Geometry: see drawing. Coordinates: mm, zero at the bounding-box minimum. Round coordinates to 2 decimals unless told otherwise and drop trailing zeros. Order: outer loops, then holes, each group sorted by start corner. A loop starts at its lowest first (then second) coordinate and runs counter-clockwise, first axis right, second up. Notation, with made-up numbers: (88.5, -22) -> (121.5, -22) arc R16 ccw to (121.5, -15) -> close; hole circle Ø11 at (53, 87.25). An arc over 180 degrees is marked (long way). Use a Markdown table: item, result.
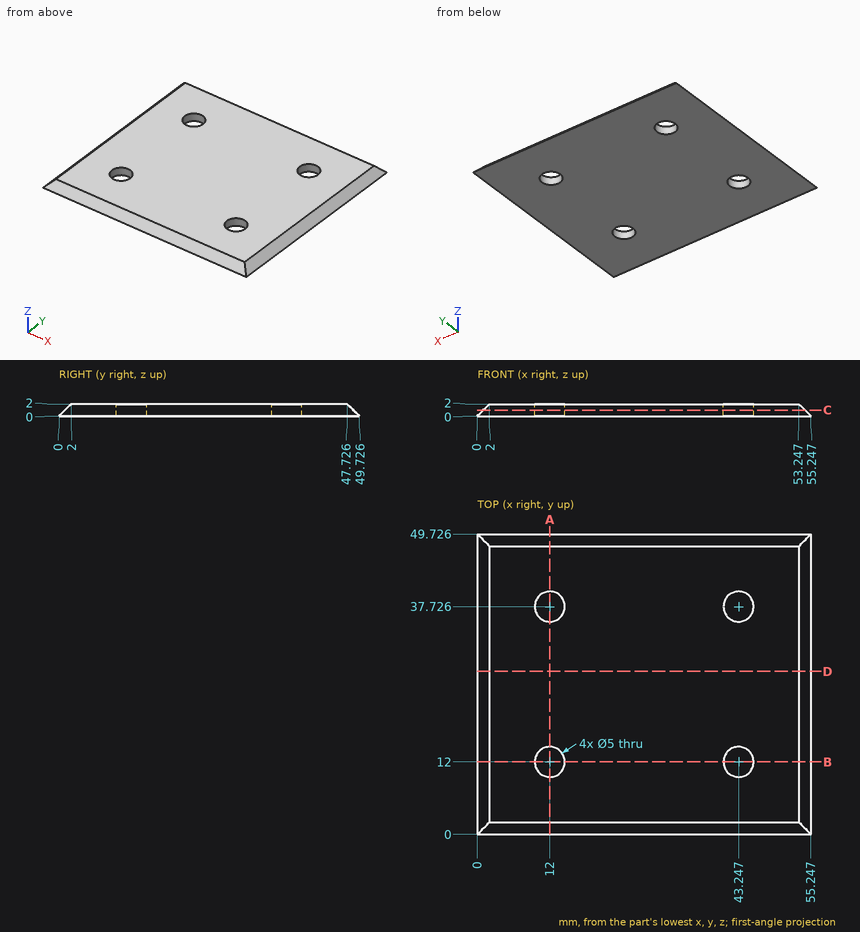
1) Ray query, probe 1 along Y at (x, z) = (12, 1.4) (1 decimal); probe 2 along Y at (x, z) = (12, 1.2) (1 decimal); probe 3 along X at (y, z) = (10, 1.35). Return the intervals inside material, ascending.
Answer key:
| item | result |
|---|---|
| probe 1 | y = 1.4 to 9.5, 14.5 to 35.2, 40.2 to 48.3 |
| probe 2 | y = 1.2 to 9.5, 14.5 to 35.2, 40.2 to 48.5 |
| probe 3 | x = 1.35 to 10.5, 13.5 to 41.75, 44.75 to 53.9 |
2) Cut plane A-A on x = 12. Return loops of the section in (y, z).
Answer key:
| item | result |
|---|---|
| outline | (0, 0) -> (9.5, 0) -> (9.5, 2) -> (2, 2) -> close; (14.5, 0) -> (35.23, 0) -> (35.23, 2) -> (14.5, 2) -> close; (40.23, 0) -> (49.73, 0) -> (47.73, 2) -> (40.23, 2) -> close |
3) Cut plane D-D on y = 27. Return loops of the section in (x, z), and give its area (4 significant figures).
Answer key:
| item | result |
|---|---|
| outline | (0, 0) -> (55.25, 0) -> (53.25, 2) -> (2, 2) -> close |
| area | 106.5 mm^2 |
4) Cut plane B-B on y = 12. Return loops of the section in (x, z), and give its area (3 significant figures).
Answer key:
| item | result |
|---|---|
| outline | (0, 0) -> (9.5, 0) -> (9.5, 2) -> (2, 2) -> close; (14.5, 0) -> (40.75, 0) -> (40.75, 2) -> (14.5, 2) -> close; (45.75, 0) -> (55.25, 0) -> (53.25, 2) -> (45.75, 2) -> close |
| area | 86.5 mm^2 |
5) Cut plane C-C on z = 1. Return loops of the section in (x, y), and give its area (3 significant figures).
Answer key:
| item | result |
|---|---|
| outline | (1, 1) -> (54.25, 1) -> (54.25, 48.73) -> (1, 48.73) -> close; hole circle Ø5 at (12, 12); hole circle Ø5 at (12, 37.73); hole circle Ø5 at (43.25, 12); hole circle Ø5 at (43.25, 37.73) |
| area | 2,460 mm^2 |
6) Contact query for a flat-ended pin moving along its axis: P1, Ø3, axis at x = 43.25, y = 37.73, coming from the +Z side (3 decimals). Output: stop coordinate, or through.
Answer key:
| item | result |
|---|---|
| P1 | passes through |
